Design review of the part built by this model. Coordinates are the model's own, in mm. Face numbers are marked on the shaded views. Round coordinates to 2 decimals unless told otherwise and drop trailing zeros. Write each loop counter-clockwise with the first axis right and the second up, starting at its lowest first coordinate (ties: lowest second). Pieces come first, ordered by that corner, then holes. Notation, with made-up numbers: M 39.25,-29 L 53.25,-29 A25 cw 53.25,10 Z; hole C 82.25,11.5 d10. An arc over 180 degrees is marked long. Use CSV: the item, a comma, the result in double quotes.
from build123d import *

# Parameters (mm, degrees)
F0_W     = 56
F0_H     = 50
F1_DEPTH = 1.2
F2_W     = 5.4
F2_H     = 13
F3_DEPTH = 1.2
F4_W     = 51
F4_H     = 43.6
F4_W_2   = 5.4
F4_H_2   = 13
F5_DEPTH = 3
F6_W     = 50
F6_H     = 42.6
F7_DEPTH = 3


with BuildPart() as f1:
    # F0 (on Top) → F1 (new body)
    with BuildSketch(Plane.XY):
        with Locations((-40.981666, -6.123801)):
            Rectangle(F0_W, F0_H)
    extrude(amount=F1_DEPTH)

    # F2 (on face) → F3 (cut)
    with BuildSketch(Plane.XY.offset(1.2)):
        with Locations((-20.466588, -11.532844)):
            Rectangle(F2_W, F2_H)
    extrude(amount=-F3_DEPTH, mode=Mode.SUBTRACT)

    # F4 (on face) → F5 (join)
    with BuildSketch(Plane.XY.offset(1.2)):
        with Locations((-40.981666, -6.123801)):
            Rectangle(F4_W, F4_H)
        with Locations((-20.466588, -11.532844)):
            Rectangle(F4_W_2, F4_H_2, mode=Mode.SUBTRACT)
    extrude(amount=F5_DEPTH)

    # F6 (on face) → F7 (cut)
    with BuildSketch(Plane.XY.offset(4.2)):
        with Locations((-40.981666, -6.123801)):
            Rectangle(F6_W, F6_H)
    extrude(amount=-F7_DEPTH, mode=Mode.SUBTRACT)


solid = f1.part
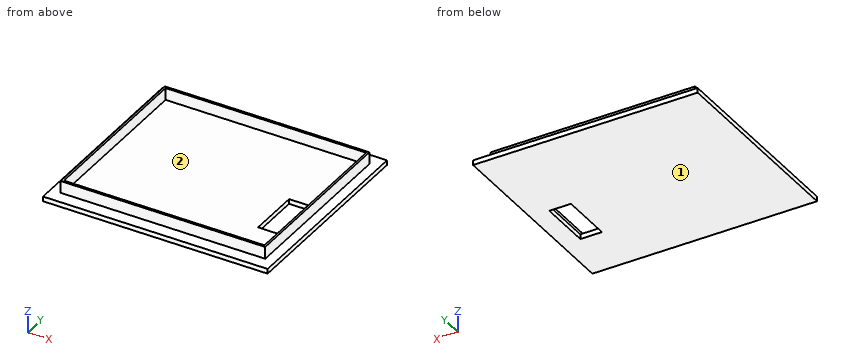
1) The part is to be moulded in two halves that separate along Y. For the marked faces 1 and 2, say which applies: released by +Y, released by -Y, zero draft, split by the parting line, or undercut.
Answers:
face 1,"zero draft"
face 2,"undercut"
2) Add section A-A on z = 2.35. Write out the cut boundary in (x, y).
Answers:
outline,"M -66.48,-27.92 L -15.48,-27.92 L -15.48,15.68 L -66.48,15.68 Z; hole M -65.98,-27.42 L -15.98,-27.42 L -15.98,15.18 L -65.98,15.18 Z"
3) Wall thickness on line 1 along X through (y, z) = (6, 4.05); line 2 along Y through (x, z) = (-45.5, 3.5); line 3 along Z through (x, y) = (-46, -19.5): over which ranges is each line inside the solid? List them lowest first. Write a range as [from, to].
Answers:
line 1,"[-66.48, -65.98], [-15.98, -15.48]"
line 2,"[-27.92, -27.42], [15.18, 15.68]"
line 3,"[0, 1.2]"
4) For pin 1 Ø1.5 at (x, z) = (-34.5, 3) entering from -Y; pin 2 Ø2.5 at (y, z) = (3, 2.5) entering from -X; pin 3 Ø25 at (x, y) = (-47.5, -14.5) entering from +Z, all flat-tipped, find the tip position at first contact; note any pin that passes through.
Answers:
pin 1,"y = -27.92"
pin 2,"x = -66.48"
pin 3,"z = 1.2"
5) Add section D-D on x = -49. Write out the cut boundary in (y, z).
Answers:
outline,"M -31.12,0 L 18.88,0 L 18.88,1.2 L 15.68,1.2 L 15.68,4.2 L 15.18,4.2 L 15.18,1.2 L -27.42,1.2 L -27.42,4.2 L -27.92,4.2 L -27.92,1.2 L -31.12,1.2 Z"
6) Add section C-C on x = -21.5. Write out the cut boundary in (y, z), then the cut area to 3 significant figures.
Answers:
outline,"M -31.12,0 L -18.03,0 L -18.03,1.2 L -27.42,1.2 L -27.42,4.2 L -27.92,4.2 L -27.92,1.2 L -31.12,1.2 Z; M -5.03,0 L 18.88,0 L 18.88,1.2 L 15.68,1.2 L 15.68,4.2 L 15.18,4.2 L 15.18,1.2 L -5.03,1.2 Z"
area,"47.4 mm²"
7) Add section B-B on y = -11. Write out the cut boundary in (x, z).
Answers:
outline,"M -68.98,0 L -23.17,0 L -23.17,1.2 L -65.98,1.2 L -65.98,4.2 L -66.48,4.2 L -66.48,1.2 L -68.98,1.2 Z; M -17.77,0 L -12.98,0 L -12.98,1.2 L -15.48,1.2 L -15.48,4.2 L -15.98,4.2 L -15.98,1.2 L -17.77,1.2 Z"
